The model under review builds one solid part; all positions refer to its coordinate system, in mm. A direction names the side the tool comes from. Round coordinates to 2 decimals unless told otherwise and drop trailing zeros. Loops run counter-clockwise (first coordinate to the right, second up) from the corner with the lowest first, then second, coordinate; pieces in that order, holes last. Notation, with made-up numbers: M -18.75,27 L 40.25,27 A20 ccw 40.25,62 Z; hole C 59,55.25 d10. An arc over 180 degrees is marked long. Use a Markdown table: item, result. Add a question column.
```python
from build123d import *

# Parameters (mm, degrees)
ESBO_O1_W                = 8
ESBO_O1_H                = 6
RESSALTO_EXTRUS_O1_DEPTH = 5.1
CORTE_EXTRUS_O1_DEPTH    = 2.4
ESBO_O3_R                = 1.875
CORTE_EXTRUS_O2_DEPTH    = 2.7


with BuildPart() as part:
    # Esboço1 → Ressalto-extrusão1 (new body)
    with BuildSketch(Plane.XY):
        Rectangle(ESBO_O1_W, ESBO_O1_H)
    extrude(amount=RESSALTO_EXTRUS_O1_DEPTH)

    # Esboço2 → Corte-extrusão1 (cut)
    with BuildSketch(Plane.XY.offset(5.1)):
        Polygon((0, -3.319764048), (2.875, -1.659882024), (2.875, 1.659882024), (0, 3.319764048), (-2.875, 1.659882024), (-2.875, -1.659882024), align=None)
    extrude(amount=-CORTE_EXTRUS_O1_DEPTH, mode=Mode.SUBTRACT)

    # Esboço3 → Corte-extrusão2 (cut)
    with BuildSketch(Plane.XY.offset(2.7)):
        Circle(ESBO_O3_R)
    extrude(amount=-CORTE_EXTRUS_O2_DEPTH, mode=Mode.SUBTRACT)


solid = part.part
```
(1) Draft analysis for pull direction Y (two halves, no side actions). For faces 1 (the face through (1.73, 2.32, 3.92)), 2 (the face through (1.7, -2.34, 3.92)), 3 (the face through (-0.1, -3, 2.5)), 4 (the face through (3.4, 0, 5.1)), state which applies: released by +Y, released by -Y, zero draft, split by the parting line, or undercut.
(2) Consider section A-A, the plane x = 0. Give the boundary of the cut face in (y, z) (3 decimals).
(3) For faces 5 (the face through (4, 0, 3)), 6 (the face through (-2.875, 0, 4)), list the 3-axis set-ups (+Z, -Z, +X, -X, +Y, -Y) from which the entire face can be reached by the end or side of a thin tool; tool diameter is ignored.
(4) Consider section D-D, the plane z = 0.75. Give the boundary of the cut face in (x, y) (3 decimals).
(5) Insertion check: pin 1 Ø1.7 at (x, y) = (0, 0.5) entering from +Z. The pin has a flat end and moves straight along its axis. Give the tip position at first contact, or say it passes through.
(6) Consider section B-B, the plane z = 4.15. Give the boundary of the cut face in (x, y) (3 decimals).
(7) Consider section C-C, the plane y = 0. Give the boundary of the cut face in (x, z) (3 decimals), then the cut area to 3 significant figures.
(8) To check wall thickness, follow probe 1 along Y at (x, z) = (0, 0.75) (3 decimals); probe 2 along X at (y, z) = (0.75, 3.65) (3 decimals); probe 3 along Z at (x, y) = (2.25, -1.5). State the ranges of each line that lie inside material, in increasing order.
Found:
| question | item | result |
|---|---|---|
| 1 | face 1 | undercut |
| 1 | face 2 | undercut |
| 1 | face 3 | released by -Y |
| 1 | face 4 | zero draft |
| 2 | outline | M -3,0 L -1.875,0 L -1.875,2.7 L -3,2.7 Z; M 1.875,0 L 3,0 L 3,2.7 L 1.875,2.7 Z |
| 3 | face 5 | +Z, -Z, +X, +Y, -Y |
| 3 | face 6 | +Z |
| 4 | outline | M -4,-3 L 4,-3 L 4,3 L -4,3 Z; hole C 0,0 d3.75 |
| 5 | pin 1 | passes through |
| 6 | outline | M -4,-3 L -0.554,-3 L -2.875,-1.66 L -2.875,1.66 L -0.554,3 L -4,3 Z; M 0.554,-3 L 4,-3 L 4,3 L 0.554,3 L 2.875,1.66 L 2.875,-1.66 Z |
| 7 | outline | M -4,0 L -1.875,0 L -1.875,2.7 L -2.875,2.7 L -2.875,5.1 L -4,5.1 Z; M 1.875,0 L 4,0 L 4,5.1 L 2.875,5.1 L 2.875,2.7 L 1.875,2.7 Z |
| 7 | area | 16.9 mm^2 |
| 8 | probe 1 | y = -3 to -1.875, 1.875 to 3 |
| 8 | probe 2 | x = -4 to -2.875, 2.875 to 4 |
| 8 | probe 3 | z = 0 to 2.7 |
